Source: CAD feature listing. Evaluate the final solid. Frame: model axes, mm. Give positions to 0.01 mm unless a question says otherwise; leave off trailing zeros. Order: outer loops, then holes, each group sorted by start corner. A loop starts at its lowest first (then second) coordinate and runs counter-clockwise, first axis right, second up. Notation, with made-up numbers: M -9.5,4 L 0.5,4 A11 cw 0.5,15 Z; hole C -5.75,16.25 d7. An arc over 180 degrees is marked long. Answer in a Markdown table with one row per item. Add a question column.
(1) Section query C-C, the plane y = 0.7. Return loops of the section in (x, z).
(2) Mould query, pull axis X, two halves, no side actions, for faces 1 (the face through (-5, 2, -6)), 2 (the face through (0.234, 2.465, 3.527)), 3 (the face through (-0.923, 2.465, -14.114)), 4 (the face through (2.3, 5, -5.1)). Classes: pulls with the +X half, pulls with the -X half, needs draft (parallel to the pull), parting line crosses it, or undercut.
(3) Section query B-B, the plane z = -14.5. Return loops of the section in (x, y).
(4) Section query A-A, the plane x = 0. Return loops of the section in (y, z).
(5) Material intervals for line 1 along Z through (x, y) = (0, 3.3); line 2 along X through (y, z) = (2.4, -10); line 3 along Z through (x, y) = (-0.75, 3.25), sorted ascending.
Autodesk Inventor part; units mm, degrees
ref_plane "YZ Plane" through (0, 0, 0) normal (1, 0, 0) x (0, 1, 0)
ref_plane "XZ Plane" through (0, 0, 0) normal (0, 1, 0) x (-1, 0, 0)
ref_plane "XY Plane" through (0, 0, 0) normal (0, 0, 1) x (1, 0, 0)
sketch "Sketch1" plane through (0, 0, 0) normal (0, 1, 0) x (-1, 0, 0)
  line L0 (-5, -21.8883) -> (5, -21.8883)
  line L1 (5, -21.8883) -> (5, 11.3117)
  line L2 (5, 11.3117) -> (-5, 11.3117)
  line L3 (-5, 11.3117) -> (-5, -21.8883)
  circle A0 centre (0, 0.1617) radius 1.85
  circle A1 centre (0, -5.0883) radius 1.9
  line L4 (0, 11.3117) -> (0, -21.8883) construction
  circle A2 centre (0, 5.3117) radius 1.8
  circle A3 centre (0, -10.4383) radius 1.95
  circle A4 centre (0, -15.8883) radius 2
  dimension "d1" = 10
  dimension "d2" = 3.7
  dimension "d3" = 3.8
  dimension "d4" = 1.5
  dimension "d5" = 3.6
  dimension "d6" = 1.5
  dimension "d8" = 3.9
  dimension "d9" = 1.5
  dimension "d10" = 4
  dimension "d11" = 1.5
  dimension "d12" = 6
  dimension "d13" = 6
extrude "Extrusion1" add sketch "Sketch1" along normal blind 5
properties part number "Test Block for Inserts"
Values follow:
| question | item | result |
|---|---|---|
| 1 | outline | M -5,-21.89 L 5,-21.89 L 5,11.31 L -5,11.31 Z; hole C 0,-15.89 d4; hole C 0,-10.44 d3.9; hole C 0,-5.09 d3.8; hole C 0,0.16 d3.7; hole C 0,5.31 d3.6 |
| 2 | face 1 | pulls with the -X half |
| 2 | face 2 | undercut |
| 2 | face 3 | undercut |
| 2 | face 4 | needs draft |
| 3 | outline | M -5,0 L -1.44,0 L -1.44,5 L -5,5 Z; M 1.44,0 L 5,0 L 5,5 L 1.44,5 Z |
| 4 | outline | M 0,-21.89 L 5,-21.89 L 5,-17.89 L 0,-17.89 Z; M 0,-13.89 L 5,-13.89 L 5,-12.39 L 0,-12.39 Z; M 0,-8.49 L 5,-8.49 L 5,-6.99 L 0,-6.99 Z; M 0,-3.19 L 5,-3.19 L 5,-1.69 L 0,-1.69 Z; M 0,2.01 L 5,2.01 L 5,3.51 L 0,3.51 Z; M 0,7.11 L 5,7.11 L 5,11.31 L 0,11.31 Z |
| 5 | line 1 | z = -21.89 to -17.89, -13.89 to -12.39, -8.49 to -6.99, -3.19 to -1.69, 2.01 to 3.51, 7.11 to 11.31 |
| 5 | line 2 | x = -5 to -1.9, 1.9 to 5 |
| 5 | line 3 | z = -21.89 to -17.74, -14.03 to -12.24, -8.64 to -6.83, -3.34 to -1.53, 1.85 to 3.68, 6.95 to 11.31 |
